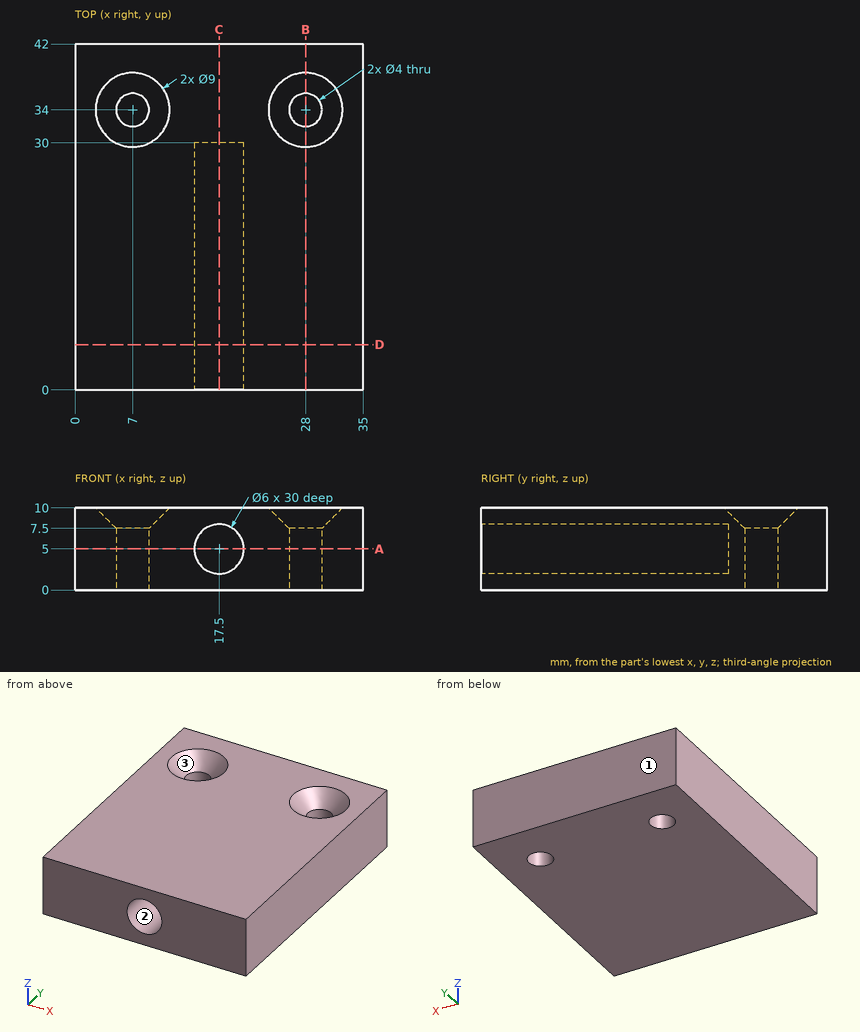
Drawing for the job (mm, zero at the part's lowest x, y, z). Give positions to 0.01 mm unless a question says otherwise; leave off trailing zeros. Order: outer loops, then holes, each group sorted by start corner. A loop starts at its lowest first (then second) coordinate and runs counter-clockwise, first axis right, second up. Notation, with made-up numbers: (56.5, 11.5) - (62.5, 11.5) arc R10 cw to (62.5, 30.5) - close; hole circle Ø9 at (-17.5, 38.25). An arc over 180 degrees is marked (long way). Use one line per item in the form item = value.
Item 1: Slice it at A-A on z = 5. Give the cut face in (x, y).
Solution:
outline = (0, 0) - (14.5, 0) - (14.5, 30) - (20.5, 30) - (20.5, 0) - (35, 0) - (35, 42) - (0, 42) - close; hole circle Ø4 at (7, 34); hole circle Ø4 at (28, 34)
Item 2: Slice it at C-C on x = 17.5. Give the cut face in (y, z), and give its area (3 significant figures).
Solution:
outline = (0, 0) - (42, 0) - (42, 10) - (0, 10) - (0, 8) - (30, 8) - (30, 2) - (0, 2) - close
area = 240 mm2
Item 3: Probe probe 1 along Y at (x, z) = (28, 5.25); probe 2 along X at (y, z) = (26, 5.25); probe 3 along X at (y, z) = (22, 3.75). List the from-to ranges inside material, lowest first. Write a range as from..to.
Solution:
probe_1 = 0..32, 36..42
probe_2 = 0..14.51, 20.49..35
probe_3 = 0..14.77, 20.23..35
Item 4: Pin check, flat tip, straight feed: pin 1 Ø3 at (y, z) = (28, 6.5) entering from -X. Stop position of the tip, or through.
Solution:
pin_1 = 0
Item 5: Slice it at B-B on x = 28. Give the cut face in (y, z).
Solution:
outline = (0, 0) - (32, 0) - (32, 7.5) - (29.5, 10) - (0, 10) - close; (36, 0) - (42, 0) - (42, 10) - (38.5, 10) - (36, 7.5) - close
Item 6: Two-plate mould, pull along Y, no slides. Class the marked faces 1, 2 and 3: released by +Y, released by -Y, zero draft, split by the parting line, or undercut.
Solution:
face_1 = released by +Y
face_2 = zero draft
face_3 = undercut
Item 7: Slice it at D-D on y = 5.5. Give the cut face in (x, z).
Solution:
outline = (0, 0) - (35, 0) - (35, 10) - (0, 10) - close; hole circle Ø6 at (17.5, 5)
